from build123d import *

# Parameters (mm, degrees)
BOSS_EXTRUDE2_DEPTH     = 4
SKETCH2_R               = 1.2
CUT_EXTRUDE2_DEPTH      = 6.5
CUT_EXTRUDE2_DEPTH_BACK = 1
SKETCH3_R               = 0.75
CUT_EXTRUDE3_DEPTH      = 5
CUT_EXTRUDE3_DEPTH_BACK = 5


with BuildPart() as part:
    # Sketch1 → Boss-Extrude2 (new body, symmetric)
    with BuildSketch(Plane.XY):
        Polygon((0, 0), (6.1, 0), (6.1, 2.6), (20.3, 2.6), (20.3, 5.5), (0, 5.5), align=None)
    extrude(amount=BOSS_EXTRUDE2_DEPTH, both=True)

    # Sketch2 → Cut-Extrude2 (cut, two sides)
    with BuildSketch(Plane(origin=(0, 0, 0), x_dir=(1, 0, 0), z_dir=(0, 1, 0))) as cut_extrude2_sk:
        with Locations((2.7, 0)):
            Circle(SKETCH2_R)
    extrude(amount=CUT_EXTRUDE2_DEPTH, mode=Mode.SUBTRACT)
    extrude(cut_extrude2_sk.sketch, amount=-CUT_EXTRUDE2_DEPTH_BACK, mode=Mode.SUBTRACT)

    # Sketch3 → Cut-Extrude3 (cut, two sides)
    with BuildSketch(Plane.XY) as cut_extrude3_sk:
        with Locations((6.85, 2.6)):
            Circle(SKETCH3_R)
    extrude(amount=CUT_EXTRUDE3_DEPTH, mode=Mode.SUBTRACT)
    extrude(cut_extrude3_sk.sketch, amount=-CUT_EXTRUDE3_DEPTH_BACK, mode=Mode.SUBTRACT)


solid = part.part
CAD build for the part. Positions are in the model's coordinates, mm. A direction names the side the tool comes from. Coordinates: 2 decimals unless noted, no trailing zeros. Order: outer loops, then holes, each group sorted by start corner. A loop starts at its lowest first (then second) coordinate and runs counter-clockwise, first axis right, second up. Notation, with made-up numbers: (88, 65) -> (106, 65) arc R16 cw to (106, 85) -> close; hole circle Ø11 at (46.25, 6.5). An arc over 180 degrees is marked (long way). Answer in a Markdown table with one row per item.
1) Flat gauge pin, fed straight in: P1, Ø1.3, axis at y = 1, z = -1, coming from the +X side. Where does the tip first touch, or does it go through?
Check values:
| item | result |
|---|---|
| P1 | x = 6.1 |
2) Band-saw the part on C-C (y = 0.7). List the corners of the cut face in (x, z), and give its area (3 significant figures).
Check values:
| item | result |
|---|---|
| outline | (0, -4) -> (6.1, -4) -> (6.1, 4) -> (0, 4) -> close; hole circle Ø2.4 at (2.7, 0) |
| area | 44.3 mm2 |
3) Drill centre lines: line 1 (Z direction, x = 2.7, y = 3.15); line 2 (X direction, y = 3.75, z = 0); line 3 (Y direction, x = 15.5, z = -3). Where is each one in solid material? Low to high.
Check values:
| item | result |
|---|---|
| line 1 | -4 to -1.2, 1.2 to 4 |
| line 2 | 0 to 1.5, 3.9 to 20.3 |
| line 3 | 2.6 to 5.5 |
4) Band-saw the part on A-A (x = 2.7). List the corners of the cut face in (y, z), and give its area (3 significant figures).
Check values:
| item | result |
|---|---|
| outline | (0, -4) -> (5.5, -4) -> (5.5, -1.2) -> (0, -1.2) -> close; (0, 1.2) -> (5.5, 1.2) -> (5.5, 4) -> (0, 4) -> close |
| area | 30.8 mm2 |
5) Band-saw the part on B-B (z = -0.25). List the corners of the cut face in (x, y).
Check values:
| item | result |
|---|---|
| outline | (0, 0) -> (1.53, 0) -> (1.53, 5.5) -> (0, 5.5) -> close; (3.87, 0) -> (6.1, 0) -> (6.1, 2.6) arc R0.75 cw to (7.6, 2.6) -> (20.3, 2.6) -> (20.3, 5.5) -> (3.87, 5.5) -> close |
6) Which spindle directions (+Z, -Z, +X, -X, +Y, -Y) get a long thin tool onto all of the face, cutting with end or side? Do faces 5 (the face through (14, 2.6, 0)), 6 (the face through (20.3, 4, 0)). Say none if no direction does.
Check values:
| item | result |
|---|---|
| face 5 | +Z, -Z, +X, -Y |
| face 6 | +Z, -Z, +X, +Y, -Y |
7) Mould opens along X. For faces 1 (the face through (3.845, 2.712, -0.36)), 2 (the face through (8, 3, 4)), 3 (the face through (6.1, 1, 0)), 4 (the face through (0, 3, 0)) say: pulls with the +X half, pulls with the -X half, needs draft (parallel to the pull), parting line crosses it, or undercut.
Check values:
| item | result |
|---|---|
| face 1 | undercut |
| face 2 | needs draft |
| face 3 | pulls with the +X half |
| face 4 | pulls with the -X half |
8) Band-saw the part on D-D (x = 6.85). List the corners of the cut face in (y, z).
Check values:
| item | result |
|---|---|
| outline | (3.35, -4) -> (5.5, -4) -> (5.5, 4) -> (3.35, 4) -> close |
